from build123d import *

# Parameters (mm, degrees)
SKETCH1_W           = 95.25
SKETCH1_H           = 95.25
BOSS_EXTRUDE1_DEPTH = 6.35
BOSS_EXTRUDE2_DEPTH = 6.35


with BuildPart() as part:
    # Sketch1 → Boss-Extrude1 (new body)
    with BuildSketch(Plane.XY):
        with Locations((-47.625, 47.625)):
            Rectangle(SKETCH1_W, SKETCH1_H)
    extrude(amount=BOSS_EXTRUDE1_DEPTH)

    # Sketch3 → Boss-Extrude2 (add)
    with BuildSketch(Plane(origin=(0, 0, 0), x_dir=(0, 0, -1), z_dir=(1, 0, 0))):
        Polygon((-6.35, 55.696344872), (-20.329979404, 63.767689744), (-34.309958807, 55.696344872), (-34.309958807, 39.553655128), (-20.329979404, 31.482310256), (-6.35, 39.553655128), align=None)
    extrude(amount=-BOSS_EXTRUDE2_DEPTH)


solid = part.part
Work out the finished part from the listing and answer in its coordinate system (mm). A direction names the side the tool comes from. Give positions to 0.01 mm unless a question says otherwise; leave off trailing zeros. Write each loop counter-clockwise with the first axis right and the second up, starting at its lowest first coordinate (ties: lowest second). Pieces come first, ordered by that corner, then holes. Notation, with made-up numbers: M -2,14.25 L 55,14.25 A20 cw 55,29.25 Z; hole C 32.25,33 d1. An arc over 180 degrees is marked long. Answer as CSV lines item,"result".
Q1. A cutting plane is placed at D-D on z = 29.5. Write down the section's boundary in (x, y).
A:
outline,"M -6.35,36.78 L 0,36.78 L 0,58.47 L -6.35,58.47 Z"
Q2. The mould has two halves that part along Z. Classify faces 1 (the flat face through (-95.25, 47, 3)), 2 (the flat face through (-3, 48, 34.31)), 3 (the flat face through (-3.131, 59.676, 13.242)), 4 (the flat face through (-48, 48, 0)): +Z half, -Z half, draft (parallel to the pull), parting line (faces both ways), or undercut.
A:
face 1,"draft"
face 2,"+Z half"
face 3,"undercut"
face 4,"-Z half"
Q3. Given P1, Ø1, axis at x = -66, y = 64, coming from the -Z side; P2, Ø8, axis at x = -49.5, y = 38, coming from the +Z side, each flat-ended and moving along its own axis, determine where each tip first touches the part or whether it passes through.
A:
P1,"stops at z = 0"
P2,"stops at z = 6.35"
Q4. A cutting plane is placed at C-C on y = 34.5. Write down the section's boundary in (x, z), plus the area to 3 significant figures.
A:
outline,"M -95.25,0 L 0,0 L 0,6.35 L -95.25,6.35 Z; M -6.35,15.1 L 0,15.1 L 0,25.56 L -6.35,25.56 Z"
area,"671 mm²"
Q5. A cutting plane is placed at B-B on x = -60. Write down the section's boundary in (y, z), plus the area to 3 significant figures.
A:
outline,"M 0,0 L 95.25,0 L 95.25,6.35 L 0,6.35 Z"
area,"605 mm²"
Q6. A cutting plane is placed at A-A on y = 59.5. Write down the section's boundary in (x, z).
A:
outline,"M -95.25,0 L 0,0 L 0,6.35 L -95.25,6.35 Z; M -6.35,12.94 L 0,12.94 L 0,27.72 L -6.35,27.72 Z"
Q7. A tool of negligible diameter and unlimited length cuts with its end or side. For faces 5 (the flat face through (-6.35, 48, 21)), 6 (the flat face through (-3.13, 35.46, 13.44)), 7 (the flat face through (0, 47, 13)), from which of +Z, -Z, +X, -X, +Y, -Y can it reach the whole face along a straight path? Write none if from no direction.
A:
face 5,"+Z, -X, +Y, -Y"
face 6,"+X, -X, -Y"
face 7,"+Z, -Z, +X, +Y, -Y"
Q8. Find the intervals of material crossed by probe 1 along Z at (x, y) = (-28.5, 14); probe 2 along X at (y, z) = (46.5, 23); probe 3 along Y at (x, z) = (-4, 22), in increasing order. Write a range as [from, to].
A:
probe 1,"z = [0, 6.35]"
probe 2,"x = [-6.35, 0]"
probe 3,"y = [32.45, 62.8]"
